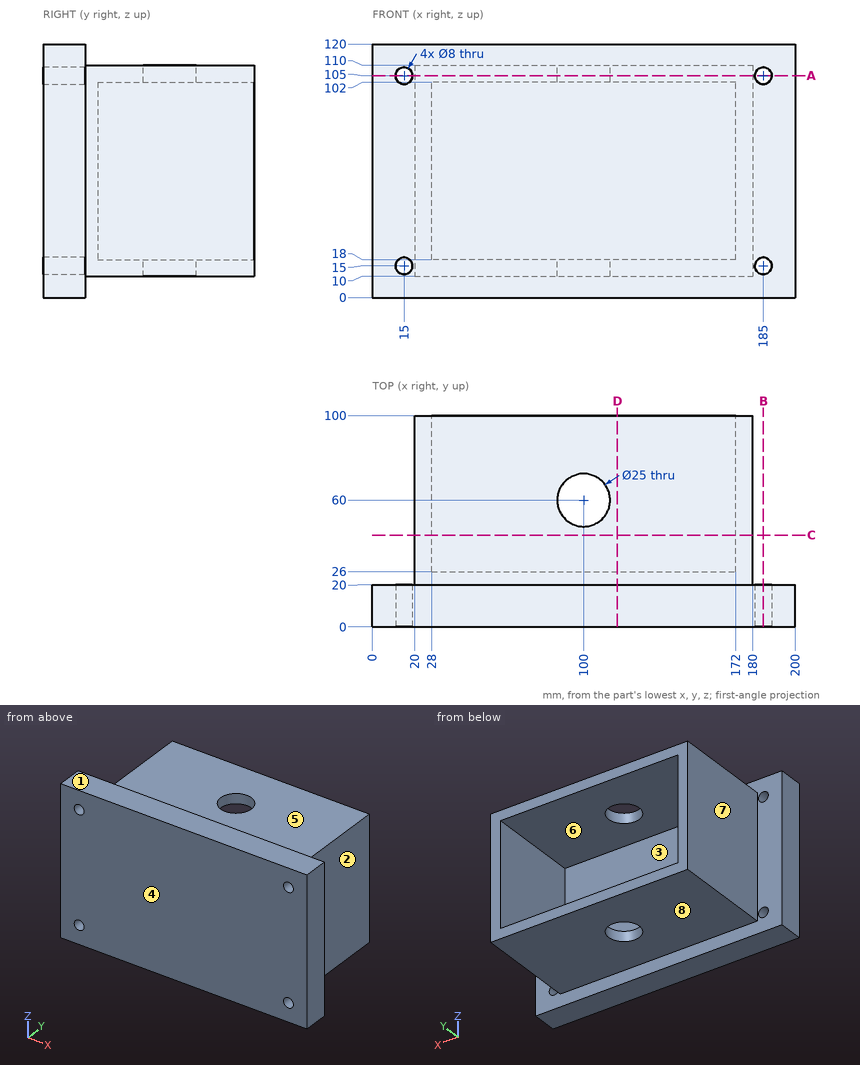
Source: three-view drawing plus pictorial views. Frame: mm from the lowest corner of the part. A direction names the side the tool comes from. Give positions to 0.01 mm unless a question says otherwise; leave off trailing zeros. Order: outer loops, then holes, each group sorted by start corner. A loop starts at its lowest first (then second) coordinate and runs counter-clockwise, first axis right, second up. Notation, with made-up numbers: (3.5, -18) -> (31.5, -18) arc R21 ccw to (31.5, 16) -> close; hole circle Ø10 at (61.25, -5). An arc over 180 degrees is marked (long way). Put each result on its own line as item: value.
Q1. Section A-A, the plane z = 105. Return loops of the section in (x, y).
Here are the results:
outline: (0, 0) -> (11, 0) -> (11, 20) -> (0, 20) -> close; (19, 0) -> (181, 0) -> (181, 20) -> (180, 20) -> (180, 100) -> (20, 100) -> (20, 20) -> (19, 20) -> close; (189, 0) -> (200, 0) -> (200, 20) -> (189, 20) -> close; hole circle Ø25 at (100, 60)
Q2. Reachability of the marked faces 1, 2, 3, 4 and 5 from +Z, -Z, +X, -X, +Y, -Y: full face, straight path, thin tool, end or side. Return the list, or none.
Here are the results:
face 1: +Z, +X, -X, +Y, -Y
face 2: +Z, -Z, +X, +Y
face 3: +Y
face 4: +Z, -Z, +X, -X, -Y
face 5: +Z, +X, -X, +Y
Q3. Section D-D, the plane x = 116. Return loops of the section in (y, z).
Here are the results:
outline: (0, 0) -> (20, 0) -> (20, 10) -> (100, 10) -> (100, 18) -> (26, 18) -> (26, 102) -> (100, 102) -> (100, 110) -> (20, 110) -> (20, 120) -> (0, 120) -> close
Q4. Material intervals for L1, parallel to X at y = 12.75, z = 105; L2, parallel to X at y = 68, z = 58; L3, parallel to Z at x = 74, y = 72.5, sorted ascending.
Here are the results:
L1: x = 0 to 11, 19 to 181, 189 to 200
L2: x = 20 to 28, 172 to 180
L3: z = 10 to 18, 102 to 110
Q5. Pin query (flat end, axial travel): pin 1 (4 mm diameter, centred on y = 50, z = 47.5, fed in from -X); pin 2 (4 mm diameter, centred on x = 100.5, y = 23.5, fed in from +Z); pin 3 (6 mm diameter, centred on x = 93, z = 97.5, fed in from +Y); pin 4 (22.5 mm diameter, centred on x = 100, y = 60, fed in from +Z). Return the tip coordinate at first contact, or that it passes through.
Here are the results:
pin 1: stops at x = 20
pin 2: stops at z = 110
pin 3: stops at y = 26
pin 4: passes through
Q6. Draft query along X for the marked faces 6, 7 and 8. Return one class per face: released by +X, released by -X, zero draft, split by the parting line, or undercut.
Here are the results:
face 6: undercut
face 7: released by -X
face 8: zero draft
Q7. Section B-B, the plane x = 185. Return loops of the section in (y, z).
Here are the results:
outline: (0, 0) -> (20, 0) -> (20, 11) -> (0, 11) -> close; (0, 19) -> (20, 19) -> (20, 101) -> (0, 101) -> close; (0, 109) -> (20, 109) -> (20, 120) -> (0, 120) -> close
Q8. Section C-C, the plane y = 43.5. Return loops of the section in (x, z).
Here are the results:
outline: (20, 10) -> (180, 10) -> (180, 110) -> (20, 110) -> close; hole (28, 18) -> (172, 18) -> (172, 102) -> (28, 102) -> close
